from build123d import *

# Parameters (mm, degrees)
F0_W     = 20
F0_H     = 20
F0_H_2   = 2100
F0_W_2   = 1300
F1_DEPTH = 20
F2_W     = 1340
F2_H     = 20
F3_DEPTH = 20
F5_DEPTH = 25
F7_DEPTH = 25


with BuildPart() as f1:
    # F0 (on Front) → F1 (new body)
    with BuildSketch(Plane.XZ):
        with Locations((-676.821301, 1047.877386)):
            Rectangle(F0_W, F0_H)
        with Locations((-676.821301, -12.122614)):
            Rectangle(F0_W, F0_H_2)
        with Locations((-16.821301, 1047.877386)):
            Rectangle(F0_W_2, F0_H)
        with Locations((-676.821301, -1072.122614)):
            Rectangle(F0_W, F0_H)
        with Locations((643.178699, 1047.877386)):
            Rectangle(F0_W, F0_H)
        with Locations((643.178699, -12.122614)):
            Rectangle(F0_W, F0_H_2)
        with Locations((-16.821301, -1072.122614)):
            Rectangle(F0_W_2, F0_H)
        with Locations((643.178699, -1072.122614)):
            Rectangle(F0_W, F0_H)
    extrude(amount=F1_DEPTH)

    # F2 (on Front) → F3 (join)
    with BuildSketch(Plane.XZ):
        with Locations((-16.821301, 522.877386)):
            Rectangle(F2_W, F2_H)
        with Locations((-16.821301, -42.122614)):
            Rectangle(F2_W, F2_H)
        with Locations((-16.821301, -627.122614)):
            Rectangle(F2_W, F2_H)
    extrude(amount=F3_DEPTH)

    # F4 (on face) → F5 (join)
    with BuildSketch(Plane(origin=(-686.821301, 0, 0), x_dir=(0, -1, 0), z_dir=(-1, 0, 0))):
        with BuildLine():
            ThreePointArc((16, -782.122614), (5.757359, -777.879974), (10, -788.122614))
            ThreePointArc((10, -788.122614), (14.242641, -786.365255), (16, -782.122614))
        make_face()
        with BuildLine():
            ThreePointArc((18, -782.122614), (4.343146, -776.46576), (10, -790.122614))
            ThreePointArc((10, -790.122614), (15.656854, -787.779469), (18, -782.122614))
        make_face()
        with BuildLine():
            ThreePointArc((16, -782.122614), (14.242641, -786.365255), (10, -788.122614))
            ThreePointArc((10, -788.122614), (5.757359, -777.879974), (16, -782.122614))
        make_face(mode=Mode.SUBTRACT)
    extrude(amount=F5_DEPTH)

    # F6 (on face) → F7 (join)
    with BuildSketch(Plane.YZ.offset(653.178699)):
        with BuildLine():
            ThreePointArc((-4, -782.122614), (-14.242641, -777.879974), (-10, -788.122614))
            ThreePointArc((-10, -788.122614), (-5.757359, -786.365255), (-4, -782.122614))
        make_face()
        with BuildLine():
            ThreePointArc((-2, -782.122614), (-15.656854, -776.46576), (-10, -790.122614))
            ThreePointArc((-10, -790.122614), (-4.343146, -787.779469), (-2, -782.122614))
        make_face()
        with BuildLine():
            ThreePointArc((-4, -782.122614), (-5.757359, -786.365255), (-10, -788.122614))
            ThreePointArc((-10, -788.122614), (-14.242641, -777.879974), (-4, -782.122614))
        make_face(mode=Mode.SUBTRACT)
    extrude(amount=F7_DEPTH)


solid = f1.part
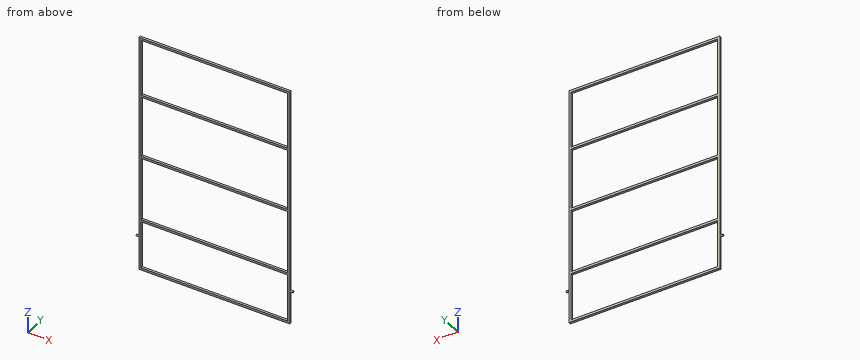
Read the model definition and answer for the solid it produces. Units are mm, in the model's axes. Coordinates: 2 decimals unless noted, no trailing zeros. Loops run counter-clockwise (first coordinate to the right, second up) from the corner with the lowest first, then second, coordinate; pieces in that order, holes last. Notation, with made-up numbers: (-20.75, -9) -> (19.25, -9) arc R9 ccw to (19.25, -3) -> close; hole circle Ø1 at (60, 23.5). An arc over 180 degrees is marked (long way). Answer in a Markdown table with one row per item.
Item 1: Straight lines are drawn through the part: line 1 along Z through (x, y) = (249, -1.25); line 2 along X through (y, z) = (-3, -552); line 3 along Z through (x, y) = (671, -10). For each, find the intervals that lie inside material, in ascending order. Write a range as [from, to].
Returned:
| item | result |
|---|---|
| line 1 | z = [-1082.12, -1062.12], [-637.12, -617.12], [-52.12, -32.12], [512.88, 532.88], [1037.88, 1057.88] |
| line 2 | x = [-686.82, -666.82], [633.18, 653.18] |
| line 3 | z = [-790.12, -788.12], [-776.12, -774.12] |
Item 2: Each of these flat-tipped pins is pushed along its axis until it touches: P1, Ø12, axis at y = -5, z = 244, coming from the +X side; P2, Ø12, axis at y = -5, z = 134.5, coming from the -X side. Where does it stop, or does it pass through?
Returned:
| item | result |
|---|---|
| P1 | stops at x = 653.18 |
| P2 | stops at x = -686.82 |
Item 3: A cutting plane is placed at A-A on x = 111.5. Determine the outline of the cut face in (y, z), plus the area to 3 significant figures.
Returned:
| item | result |
|---|---|
| outline | (-20, -1082.12) -> (0, -1082.12) -> (0, -1062.12) -> (-20, -1062.12) -> close; (-20, -637.12) -> (0, -637.12) -> (0, -617.12) -> (-20, -617.12) -> close; (-20, -52.12) -> (0, -52.12) -> (0, -32.12) -> (-20, -32.12) -> close; (-20, 512.88) -> (0, 512.88) -> (0, 532.88) -> (-20, 532.88) -> close; (-20, 1037.88) -> (0, 1037.88) -> (0, 1057.88) -> (-20, 1057.88) -> close |
| area | 2,000 mm^2 |
Item 4: A cutting plane is placed at B-B on z = 176. Determine the outline of the cut face in (x, y), plus the area to 3 significant figures.
Returned:
| item | result |
|---|---|
| outline | (-686.82, -20) -> (-666.82, -20) -> (-666.82, 0) -> (-686.82, 0) -> close; (633.18, -20) -> (653.18, -20) -> (653.18, 0) -> (633.18, 0) -> close |
| area | 800 mm^2 |
